Autodesk Inventor part; units mm, degrees
ref_plane "YZ Plane" through (0, 0, 0) normal (1, 0, 0) x (0, 1, 0)
ref_plane "XZ Plane" through (0, 0, 0) normal (0, 1, 0) x (-1, 0, 0)
ref_plane "XY Plane" through (0, 0, 0) normal (0, 0, 1) x (1, 0, 0)
sketch "Sketch1" plane through (0, 0, 0) normal (0, 0, 1) x (1, 0, 0)
  circle A0 centre (0, 0) radius 2.4 construction
  line L0 (-0.8, 2.2627) -> (-0.8, 0.8)
  line L1 (-0.8, 0.8) -> (-2.2627, 0.8)
  line L2 (-2.2627, -0.8) -> (-0.8, -0.8)
  line L3 (-0.8, -0.8) -> (-0.8, -2.2627)
  line L4 (0.8, -2.2627) -> (0.8, -0.8)
  line L5 (0.8, -0.8) -> (2.2627, -0.8)
  line L6 (2.2627, 0.8) -> (0.8, 0.8)
  line L7 (0.8, 0.8) -> (0.8, 2.2627)
  arc A1 (0.8, 2.2627) -> (-0.8, 2.2627) centre (0, 0) ccw
  arc A2 (-2.2627, 0.8) -> (-2.2627, -0.8) centre (0, 0) ccw
  arc A3 (-0.8, -2.2627) -> (0.8, -2.2627) centre (0, 0) ccw
  arc A4 (2.2627, -0.8) -> (2.2627, 0.8) centre (0, 0) ccw
  dimension "d0" = 4.8
  dimension "d1" = 1.6
extrude "Extrusion1" add sketch "Sketch1" along normal mid plane 32
sketch "Sketch2" plane through (0, 0, -16) normal (0, 0, -1) x (-1, 0, 0)
  line L0 (0.8, 0.8) -> (0.8, 2.2627)
  arc A0 (0.8, 2.2627) -> (-0.8, 2.2627) centre (0, 0) ccw
  line L1 (-0.8, 2.2627) -> (-0.8, 0.8)
  line L2 (-0.8, 0.8) -> (-2.2627, 0.8)
  arc A1 (-2.2627, 0.8) -> (-2.2627, -0.8) centre (0, 0) ccw
  line L3 (-2.2627, -0.8) -> (-0.8, -0.8)
  line L4 (-0.8, -0.8) -> (-0.8, -2.2627)
  arc A2 (-0.8, -2.2627) -> (0.8, -2.2627) centre (0, 0) ccw
  line L5 (0.8, -2.2627) -> (0.8, -0.8)
  line L6 (0.8, -0.8) -> (2.2627, -0.8)
  arc A3 (2.2627, -0.8) -> (2.2627, 0.8) centre (0, 0) ccw
  line L7 (2.2627, 0.8) -> (0.8, 0.8)
  circle A4 centre (0, 0) radius 3.2
  dimension "d7" = 6.4
extrude "Extrusion2" add sketch "Sketch2" against normal blind 0.8
fillet "Fillet1" radius 0.4 4 edges at (0, 2.4, 16) (-2.4, 0, 16) (0, -2.4, 16) (2.4, 0, 16)
fillet "Fillet1" radius 0.1 2 edges at (3.2, 0, -15.2) (3.2, 0, -16)
equation "\"d0\" = kd"
equation "\"d1\" = axlet"
equation "\"d2\" = 4 * lu"
equation "\"d7\" = tsd"
equation "\"d8\" = tsl"
equation "\"d4\" = tf"
equation "\"d10\" = lf"
properties part number "87083-DkBluishGray" material "ABS Plastic"
Source: CAD feature listing. Evaluate the final solid. Frame: model axes, mm. A direction names the side the tool comes from. Coordinates: 2 decimals unless noted, no trailing zeros. Write each loop counter-clockwise with the first axis right and the second up, starting at its lowest first coordinate (ties: lowest second). Pieces come first, ordered by that corner, then holes. Notation, with made-up numbers: (-26, -26.5) - (26, -26.5) arc R20 cw to (26, 9.5) - close; hole circle Ø9 at (13, -7). An arc over 180 degrees is marked (long way). Answer as a JSON object with one key per item and string values.
Q1. Section query A-A, the plane x = 0. Output: boundary loops of the cut face in (y, z).
Ans:
{"outline": "(-3.2, -15.9) arc R0.1 ccw to (-3.1, -16) - (3.1, -16) arc R0.1 ccw to (3.2, -15.9) - (3.2, -15.3) arc R0.1 ccw to (3.1, -15.2) - (2.4, -15.2) - (2.4, 15.6) arc R0.4 ccw to (2, 16) - (-2, 16) arc R0.4 ccw to (-2.4, 15.6) - (-2.4, -15.2) - (-3.1, -15.2) arc R0.1 ccw to (-3.2, -15.3) - close"}
Q2. First-contact query: pin 1 Ø1.2 at (x, z) = (1.5, -1.5) entering from +Y; pin 2 Ø1.6 at (y, z) = (-1.5, 1) entering from -X; pin 3 Ø3 at (x, y) = (-1, 2) entering from +Z; pin 4 Ø1 at (y, z) = (-2, -8.5) entering from +X. Flat tips, straight axial feed; report the tip coordinate or a pass-through.
Ans:
{"pin 1": "stops at y = 0.8", "pin 2": "stops at x = -2.3", "pin 3": "stops at z = 16", "pin 4": "stops at x = 0.8"}
Q3. Set-up query: faces 1 (the flat face through (-0.8, 2, 0)), 2 (the flat face through (-0.8, -2, 0)), 3 (the cylindrical face through (0, -2.4, 0)), 4 (the cylindrical face through (0, 2.4, 0)). Return all of +Z, -Z, +X, -X, +Y, -Y with unobstructed straight access to the full face (end or side cutting, diameter ignored); none if empty.
Ans:
{"face 1": "+Z, -X, +Y", "face 2": "+Z, -X, -Y", "face 3": "+Z, -Y", "face 4": "+Z, +Y"}
Q4. Draft query along Z for faces 5 (the cylindrical face through (2.539, -1.947, -15.604)), 6 (the flat face through (0, 0, -16)), 7 (the flat face through (0, 0, 16)). Return one class per face: released by +Z, released by -Z, zero draft, split by the parting line, or undercut.
Ans:
{"face 5": "zero draft", "face 6": "released by -Z", "face 7": "released by +Z"}
Q5. Section query C-C, the plane z = 8.5. Output: boundary loops of the cut face in (x, y).
Ans:
{"outline": "(-2.26, -0.8) - (-0.8, -0.8) - (-0.8, -2.26) arc R2.4 ccw to (0.8, -2.26) - (0.8, -0.8) - (2.26, -0.8) arc R2.4 ccw to (2.26, 0.8) - (0.8, 0.8) - (0.8, 2.26) arc R2.4 ccw to (-0.8, 2.26) - (-0.8, 0.8) - (-2.26, 0.8) arc R2.4 ccw to start"}
Q6. Material intervals for line 1 (X direction, y = -1.5, z = 13); line 2 (Y direction, x = 0, z = -10); line 3 (Z direction, x = 2, y = 0.5), sorted ascending. Write a range as [from, to].
Ans:
{"line 1": "x = [-0.8, 0.8]", "line 2": "y = [-2.4, 2.4]", "line 3": "z = [-16, 16]"}
